Input: part model. Units: mm. Frame: model coordinates. Face numbers are marked on the shaded views. A direction names the side the tool comes from. Give positions to 0.01 mm unless a question says otherwise; leave off trailing zeros. Order: outer loops, then holes, each group sorted by start corner. A loop starts at its lowest first (then second) coordinate and runs counter-clockwise, first axis right, second up. Notation, with made-up numbers: M -13.5,78.25 L 15.5,78.25 A18 ccw 15.5,89.25 Z; hole C 57,68 d7. An arc over 180 degrees is marked long. Use a Markdown table: item, result.
from build123d import *

# Parameters (mm, degrees)
F0_W     = 203.2
F0_H     = 192.284051628
F1_DEPTH = 25.4
F2_R     = 76.2
F3_DEPTH = 2.54
F4_W     = 76.2
F4_H     = 76.2
F5_DEPTH = 2.54
F7_DEPTH = 7.62
F8_DEPTH = 18


with BuildPart() as f1:
    # F0 (on Top) → F1 (new body)
    with BuildSketch(Plane.XY):
        with Locations((0.6476622075, -2.2640712559)):
            Rectangle(F0_W, F0_H)
    extrude(amount=F1_DEPTH)

    # F2 (on face) → F3 (cut)
    with BuildSketch(Plane.XY.offset(25.4)):
        Circle(F2_R)
    extrude(amount=-F3_DEPTH, mode=Mode.SUBTRACT)

    # F4 (on face) → F5 (join)
    with BuildSketch(Plane.XY.offset(22.86)):
        Rectangle(F4_W, F4_H)
    extrude(amount=F5_DEPTH)

    # F6 (on face) → F7 (cut)
    with BuildSketch(Plane.XY.offset(25.4)):
        Polygon((20.2086176723, -14.6824201711), (20.2086176723, 14.6824201711), (-7.7190050852, 23.756654874), (-24.9792251743, 0), (-7.7190050852, -23.756654874), align=None)
    extrude(amount=-F7_DEPTH, mode=Mode.SUBTRACT)

    # F8 (add): a face of the model
    f8_faces = [f1.faces().sort_by_distance(p)[0] for p in [
        (0, 37.0223692655, 25.4),
    ]]
    extrude(f8_faces, amount=F8_DEPTH)


solid = f1.part
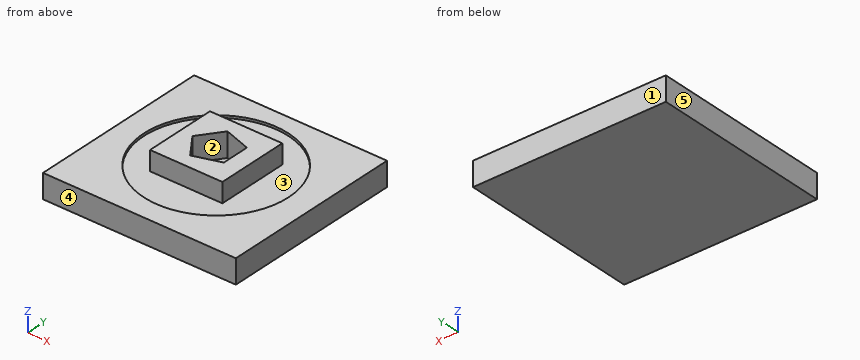
1) Cut plane D-D on y = 51.5. Return loops of the section in (x, z), and give its area (3 significant figures).
Response values:
| item | result |
|---|---|
| outline | M -100.95,0 L 102.25,0 L 102.25,25.4 L 56.16,25.4 L 56.16,22.86 L -56.16,22.86 L -56.16,25.4 L -100.95,25.4 Z |
| area | 4,880 mm² |
2) Cut plane B-B on x = -29.5. Return loops of the section in (y, z).
Response values:
| item | result |
|---|---|
| outline | M -98.41,0 L 93.88,0 L 93.88,25.4 L 70.26,25.4 L 70.26,22.86 L 38.1,22.86 L 38.1,43.4 L -38.1,43.4 L -38.1,22.86 L -70.26,22.86 L -70.26,25.4 L -98.41,25.4 Z |
3) Mould query, pull axis X, two halves, no side actions, for the marked faces 3, 4 and 5. Classes: released by +X, released by -X, zero draft, split by the parting line, or undercut.
Response values:
| item | result |
|---|---|
| face 3 | undercut |
| face 4 | zero draft |
| face 5 | released by -X |
4) Cut plane A-A on y = 21. Return loops of the section in (x, z).
Response values:
| item | result |
|---|---|
| outline | M -100.95,0 L 102.25,0 L 102.25,25.4 L 73.25,25.4 L 73.25,22.86 L 38.1,22.86 L 38.1,43.4 L 0.77,43.4 L 0.77,17.78 L -9.72,17.78 L -9.72,43.4 L -38.1,43.4 L -38.1,22.86 L -73.25,22.86 L -73.25,25.4 L -100.95,25.4 Z |
5) Cut plane C-C on x = -66.5. Return loops of the section in (y, z), and give its area (3 significant figures).
Response values:
| item | result |
|---|---|
| outline | M -98.41,0 L 93.88,0 L 93.88,25.4 L 37.2,25.4 L 37.2,22.86 L -37.2,22.86 L -37.2,25.4 L -98.41,25.4 Z |
| area | 4,700 mm² |
6) Material intervals for line 1 (Y direction, x = 0, z = 24); line 2 (Z direction, x = -43, y = 24); line 3 (Y direction, x = -15.5, z = 20), sorted ascending. Write a range as from..to.
Response values:
| item | result |
|---|---|
| line 1 | y = -98.41..-76.2, -38.1..-21.25, 21.25..38.1, 76.2..93.88 |
| line 2 | z = 0..22.86 |
| line 3 | y = -98.41..-13.05, 13.05..93.88 |
7) Reachability of the marked faces 1 and 2 from +Z, -Z, +X, -X, +Y, -Y: full face, straight path, thin tool, end or side. Return the list, or none.
Response values:
| item | result |
|---|---|
| face 1 | +Z, -Z, +X, -X, +Y |
| face 2 | +Z |
8) First-contact query: pin 1 Ø6 at (x, z) = (3, 30) entering from -Y; pin 2 Ø16.5 at (y, z) = (8, 34.5) entering from +X; pin 3 Ø10.5 at (y, z) = (1, 35.5) entering from -X. Flat tips, straight axial feed; report the tip coordinate or a pass-through.
Response values:
| item | result |
|---|---|
| pin 1 | stops at y = -38.1 |
| pin 2 | stops at x = 38.1 |
| pin 3 | stops at x = -38.1 |
